Source: CAD feature listing. Evaluate the final solid. Frame: model axes, mm. Round coordinates to 2 decimals unless told otherwise and drop trailing zeros. Loops run counter-clockwise (first coordinate to the right, second up) from the corner with the lowest first, then second, coordinate; pieces in that order, holes last. Notation, with made-up numbers: (16, 36) - (53, 36) arc R20 cw to (53, 51) - close; hole circle Ø10 at (63.5, -1). An arc over 180 degrees is marked (long way). One line per question, with ' | ' between items.
from build123d import *

# Parameters (mm, degrees)
SKETCH_1_R          = 5
EXTRUDE_1_DEPTH     = 3
SKETCH_2_R          = 2.5
CUT_EXTRUDE_1_DEPTH = 131.896905999


with BuildPart() as part:
    # 草图1 → 凸台-拉伸1 (new body)
    with BuildSketch(Plane(origin=(0, 0, 0), x_dir=(1, 0, 0), z_dir=(0, 1, 0))):
        with BuildLine():
            Line((0, -15), (120.415586748, -9.991360651))
            ThreePointArc((120.415586748, -9.991360651), (130, 0), (120.415586748, 9.991360651))
            Line((120.415586748, 9.991360651), (0, 15))
            ThreePointArc((0, 15), (-15, 0), (0, -15))
        make_face()
        with Locations(Location((0, 0, 0), (0, 0, 270))):
            Circle(SKETCH_1_R, mode=Mode.SUBTRACT)
    extrude(amount=EXTRUDE_1_DEPTH)

    # 草图2 → 切除-拉伸1 (cut, through all)
    with BuildSketch(Plane(origin=(0, 3, 0), x_dir=(1, 0, 0), z_dir=(0, 1, 0))):
        with Locations(Location((120, 0, 0), (0, 0, 270))):
            Circle(SKETCH_2_R)
    extrude(amount=-CUT_EXTRUDE_1_DEPTH, mode=Mode.SUBTRACT)


solid = part.part
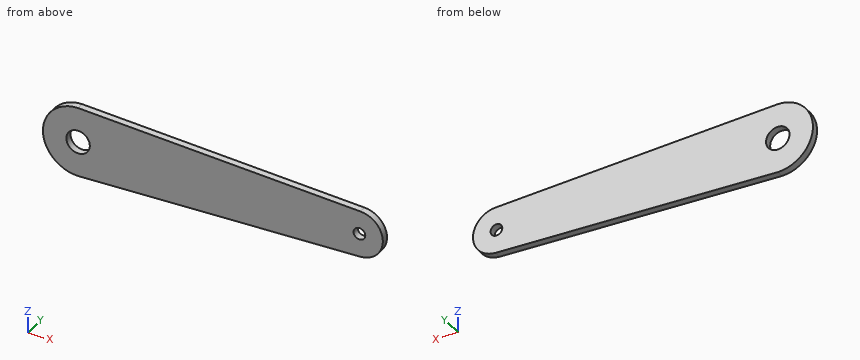
1. Contact query for flat-ended pins moving along their axis: P1, Ø1, axis at x = 98.5, y = 0.5, coming from the -Z side; P2, Ø1.5, axis at x = 29, y = 2, coming from the -Z side. Output: stop coordinate, or through.
Worked out:
P1: stops at z = -10.92 | P2: stops at z = -13.82
2. Section query B-B, the plane y = 0.75. Return loops of the section in (x, z), plus the area to 3 significant figures.
Worked out:
outline: (0, -15) - (120.42, -9.99) arc R10 ccw to (120.42, 9.99) - (0, 15) arc R15 ccw to start; hole circle Ø10 at (0, 0); hole circle Ø5 at (120, 0) | area: 3,410 mm2
3. Section query A-A, the plane z = 0. Return loops of the section in (x, y), plus the area to 3 significant figures.
Worked out:
outline: (-15, 0) - (-5, 0) - (-5, 3) - (-15, 3) - close; (5, 0) - (117.5, 0) - (117.5, 3) - (5, 3) - close; (122.5, 0) - (130, 0) - (130, 3) - (122.5, 3) - close | area: 390 mm2
4. Material intervals for probe 1 along X at (y, z) = (1.8, 0); probe 2 along X at (y, z) = (2.2, 1); probe 3 along X at (y, z) = (2.75, 4.5), sorted ascending.
Worked out:
probe 1: x = -15 to -5, 5 to 117.5, 122.5 to 130 | probe 2: x = -14.97 to -4.9, 4.9 to 117.71, 122.29 to 129.95 | probe 3: x = -14.31 to -2.18, 2.18 to 128.93
5. Section query D-D, the plane x = 77.5. Return loops of the section in (y, z).
Worked out:
outline: (0, -11.78) - (3, -11.78) - (3, 11.78) - (0, 11.78) - close
6. Section query C-C, the plane z = -12.75. Return loops of the section in (x, y), plus the area to 3 significant figures.
Worked out:
outline: (-7.9, 0) - (54.09, 0) - (54.09, 3) - (-7.9, 3) - close | area: 186 mm2
